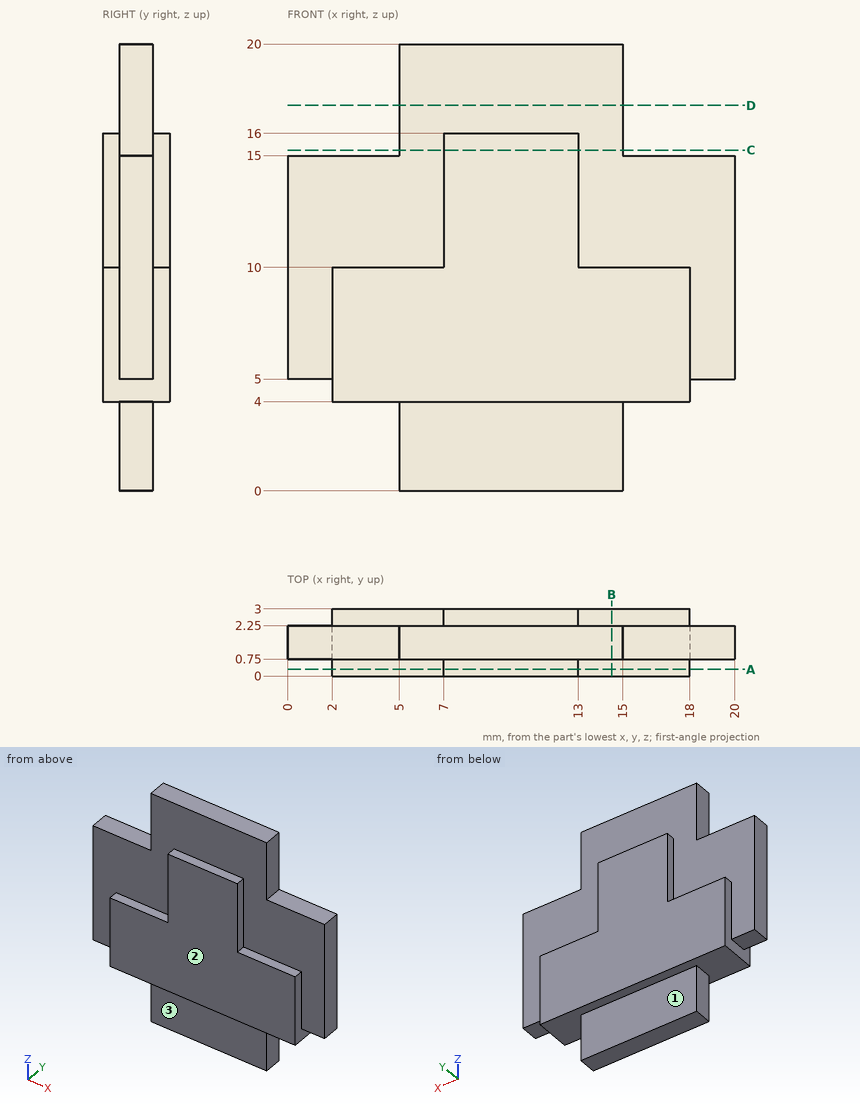
Job drawing, mm, ordinate dimensions from the low corner. One solid piece. A direction names the side the tool comes from. Round coordinates to 2 decimals unless told otherwise and drop trailing zeros. Order: outer loops, then holes, each group sorted by start corner. A loop starts at its lowest first (then second) coordinate and runs counter-clockwise, first axis right, second up. Notation, with made-up numbers: (-26, 6) - (-8, 6) arc R19 cw to (-8, 24) - close; hole circle Ø7 at (43.5, 53). An arc over 180 degrees is marked (long way). Use CSV: the item, a comma, the result in double quotes. Start each with the question number.
1) Wall check: L1, parallel to X at y = 0.5, z = 15; L2, parallel to X at y = 1.5, z = 19.25; L3, parallel to Z at x = 2.5, y = 2.55. Give the ranges that are in metal, low to high. Write a range as [from, to].
2) Saw through at B-B (x = 14.5). List the corners of the cut face in (y, z).
3) Tool access for the marked faces 1, 2 and 3: list every direction of +Z, -Z, +X, -X, +Y, -Y with a clear straight run to the whole face (end or side of a thin tool).
4) Saw through at A-A (y = 0.3). List the corners of the cut face in (x, z), and give its area (3 significant figures).
5) Saw through at D-D (z = 17.25). List the corners of the cut face in (x, y).
6) Pin check, flat tips, straight feed: pin 1 Ø0.6 at (x, y) = (15.5, 2.5) entering from +Z; pin 2 Ø0.8 at (y, z) = (1.5, 3) entering from +X; pin 3 Ø1.6 at (x, y) = (18.5, 1.5) entering from -Z. Stop position of each tip, or through.
7) Saw through at C-C (z = 15.25). List the corners of the cut face in (x, y).
Values follow:
1,L1,"x = [7, 13]"
1,L2,"x = [5, 15]"
1,L3,"z = [4, 10]"
2,outline,"(0, 4) - (0.75, 4) - (0.75, 0) - (2.25, 0) - (2.25, 4) - (3, 4) - (3, 10) - (2.25, 10) - (2.25, 20) - (0.75, 20) - (0.75, 10) - (0, 10) - close"
3,face 1,"-Z, +X, -X, +Y"
3,face 2,"+Z, -Z, +X, -X, -Y"
3,face 3,"-Z, +X, -X, -Y"
4,outline,"(2, 4) - (18, 4) - (18, 10) - (13, 10) - (13, 16) - (7, 16) - (7, 10) - (2, 10) - close"
4,area,"132 mm2"
5,outline,"(5, 0.75) - (15, 0.75) - (15, 2.25) - (5, 2.25) - close"
6,pin 1,"stops at z = 15"
6,pin 2,"stops at x = 15"
6,pin 3,"stops at z = 4"
7,outline,"(5, 0.75) - (7, 0.75) - (7, 0) - (13, 0) - (13, 0.75) - (15, 0.75) - (15, 2.25) - (13, 2.25) - (13, 3) - (7, 3) - (7, 2.25) - (5, 2.25) - close"
